Can you work these out from the drawing? Everything is in mm from the part's minimum corner. Coordinates: 2 decimals unless noted, no trailing zeros. Loops run counter-clockwise (first coordinate to the right, second up) from the corner with the lowest first, then second, coordinate; pieces in that order, holes last. Notation, with made-up numbers: M 3,52.5 L 59,52.5 A19 cw 59,85.5 Z; hole C 77.25,37.5 d10. An arc over 180 degrees is marked long. Use CSV: the item, a comma, the result in double quotes. Start each with the question number.
Q1. If we section it at A-A (z = 16): Please give me the cut outline in (x, y).
Q2. If we mould it in two halves opening along X, with no side actions, what happens to the marked faces 1, 2 and 3? For each: +X half, -X half, draft (parallel to the pull), parting line (faces both ways), or undercut.
Q3. For pin 1 Ø2 at (x, y) = (11, 2.5) entering from -Z; pin 2 Ø1.5 at (x, y) = (28.5, 1.5) entering from -Z; pin 3 Ø1.5 at (x, y) = (12.5, 1.5) entering from -Z, each with a flat end and sliding along its axis, tell me the tip position at first contact or that it passes through.
Q4. Please list where these lines run through material, in increasing order: probe 1 along X at (y, z) = (2.5, 16); probe 2 along Z at (x, y) = (17, 3.65). Write a range as [from, to].
Q5. If we section it at B-B (x = 16): Please give me the cut outline in (y, z), and give its area (4 significant figures).
Q6. If we section it at C-C (y = 3.4): Please give me the cut outline in (x, z), and give its area (3 significant figures).
Q7. If we section it at D-D (x = 20): Please give me the cut outline in (y, z), and give its area (3 significant figures).
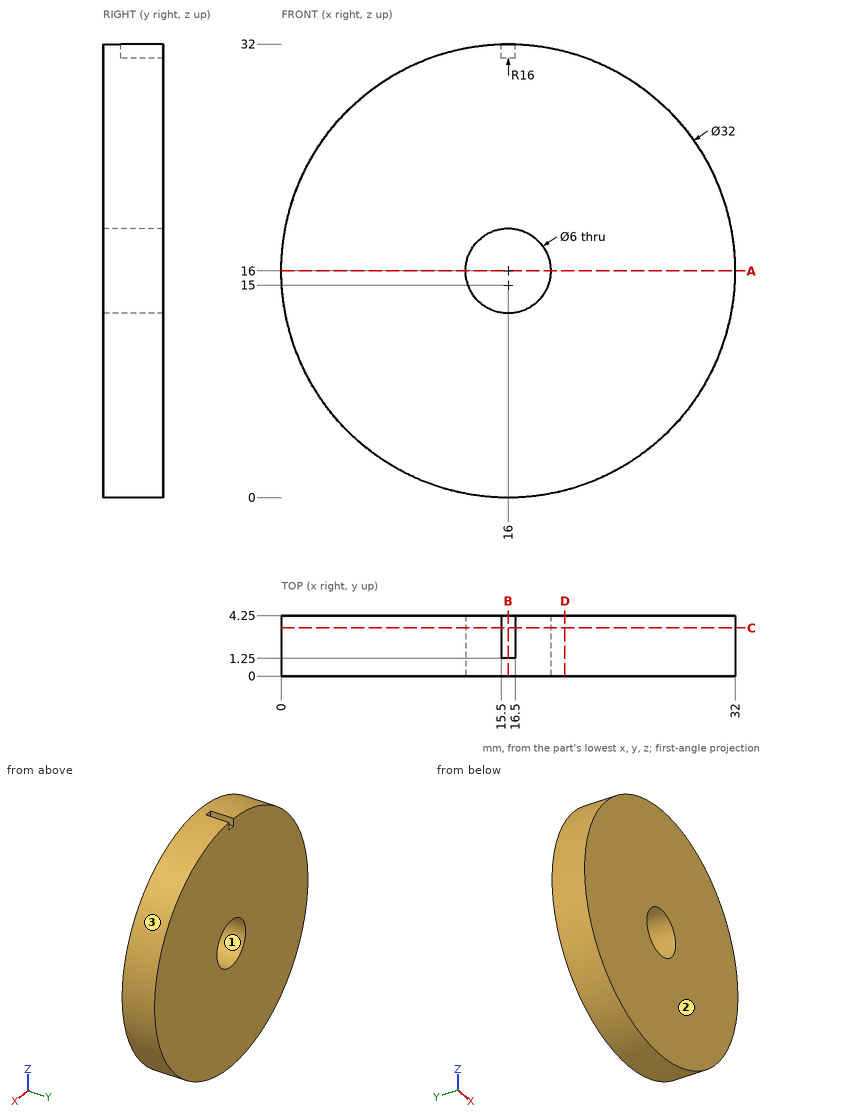
Results below:
1,outline,"M 0,0 L 13,0 L 13,4.25 L 0,4.25 Z; M 19,0 L 32,0 L 32,4.25 L 19,4.25 Z"
2,face 1,"undercut"
2,face 2,"draft"
2,face 3,"parting line"
3,pin 1,"z = 0.51"
3,pin 2,"z = 5.14"
3,pin 3,"z = 0.24"
4,probe 1,"[0, 13], [19, 32]"
4,probe 2,"[0.03, 13.17], [18.83, 31.97]"
5,outline,"M 0,0 L 4.25,0 L 4.25,13 L 0,13 Z; M 0,19 L 4.25,19 L 4.25,31 L 1.25,31 L 1.25,32 L 0,32 Z"
5,area,"107.5 mm^2"
6,outline,"M 15.5,30.99 L 15.5,31.99 A16 ccw long 16.5,31.99 L 16.5,30.99 A16 ccw Z; hole C 16,16 d6"
6,area,"775 mm^2"
7,outline,"M 0,0.51 L 4.25,0.51 L 4.25,31.49 L 0,31.49 Z"
7,area,"132 mm^2"
